Build history of the part. All positions in model axes, mm. Face numbers are marked on the shaded views. A direction names the side the tool comes from. Give positions to 0.01 mm unless a question says otherwise; leave off trailing zeros. Write each loop counter-clockwise with the first axis right and the second up, starting at its lowest first coordinate (ties: lowest second). Pieces come first, ordered by that corner, then holes. Notation, with made-up numbers: (2.25, 83) -> (28.25, 83) arc R21 ccw to (28.25, 109) -> close; hole circle Ø4 at (68, -30). An arc over 180 degrees is marked (long way). Put each result on its own line as item: value.
from build123d import *

# Parameters (mm, degrees)
SKETCH1_W           = 126
SKETCH1_H           = 68
BOSS_EXTRUDE1_DEPTH = 40
SKETCH2_W           = 117
SKETCH2_H           = 59
CUT_EXTRUDE1_DEPTH  = 38
SKETCH3_W           = 126
SKETCH3_H           = 68
SKETCH3_W_2         = 117.4
SKETCH3_H_2         = 59.4
CUT_EXTRUDE2_DEPTH  = 38
SKETCH4_R           = 10
CUT_EXTRUDE3_DEPTH  = 38
SKETCH6_R           = 1.6
CUT_EXTRUDE4_DEPTH  = 41


with BuildPart() as part:
    # Sketch1 → Boss-Extrude1 (new body)
    with BuildSketch(Plane(origin=(0, 0, 0), x_dir=(1, 0, 0), z_dir=(0, 1, 0))):
        Rectangle(SKETCH1_W, SKETCH1_H)
    extrude(amount=BOSS_EXTRUDE1_DEPTH)

    # Sketch2 → Cut-Extrude1 (cut)
    with BuildSketch(Plane(origin=(0, 40, 0), x_dir=(1, 0, 0), z_dir=(0, 1, 0))):
        Rectangle(SKETCH2_W, SKETCH2_H)
    extrude(amount=-CUT_EXTRUDE1_DEPTH, mode=Mode.SUBTRACT)

    # Sketch3 → Cut-Extrude2 (cut)
    with BuildSketch(Plane.XZ):
        Rectangle(SKETCH3_W, SKETCH3_H)
        Rectangle(SKETCH3_W_2, SKETCH3_H_2, mode=Mode.SUBTRACT)
    extrude(amount=-CUT_EXTRUDE2_DEPTH, mode=Mode.SUBTRACT)

    # Sketch4 → Cut-Extrude3 (cut)
    with BuildSketch(Plane.ZY.offset(63)):
        with Locations((0, 40)):
            Circle(SKETCH4_R)
    extrude(amount=-CUT_EXTRUDE3_DEPTH, mode=Mode.SUBTRACT)

    # Sketch6 → Cut-Extrude4 (cut, through all)
    with BuildSketch(Plane.XZ):
        with Locations((61, 15)):
            Circle(SKETCH6_R)
        with Locations((-61, 18)):
            Circle(SKETCH6_R)
        with Locations((-61, -18)):
            Circle(SKETCH6_R)
        with Locations((61, -15)):
            Circle(SKETCH6_R)
        with Locations((-21, 32)):
            Circle(SKETCH6_R)
        with Locations((-21, -32)):
            Circle(SKETCH6_R)
        with Locations((29, 32)):
            Circle(SKETCH6_R)
        with Locations((29, -32)):
            Circle(SKETCH6_R)
    extrude(amount=-CUT_EXTRUDE4_DEPTH, mode=Mode.SUBTRACT)


solid = part.part
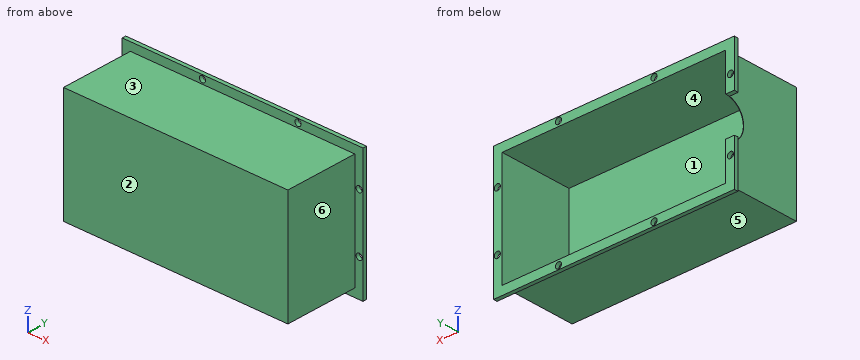
1) Slice it at D-D (x = -61). Write the cut outline in (y, z), plus the area to 3 significant figures.
Filled sheet:
outline: (38, -34) -> (40, -34) -> (40, -19.6) -> (38, -19.6) -> close; (38, -16.4) -> (40, -16.4) -> (40, -10) arc R10 cw to (38, -9.8) -> close; (38, 9.8) arc R10 cw to (40, 10) -> (40, 16.4) -> (38, 16.4) -> close; (38, 19.6) -> (40, 19.6) -> (40, 34) -> (38, 34) -> close
area: 83.5 mm2
2) Slice it at B-B (x = -21). Write the cut outline in (y, z).
Filled sheet:
outline: (0, -29.7) -> (38, -29.7) -> (38, -30.4) -> (40, -30.4) -> (40, -29.5) -> (2, -29.5) -> (2, 29.5) -> (40, 29.5) -> (40, 30.4) -> (38, 30.4) -> (38, 29.7) -> (0, 29.7) -> close; (38, -34) -> (40, -34) -> (40, -33.6) -> (38, -33.6) -> close; (38, 33.6) -> (40, 33.6) -> (40, 34) -> (38, 34) -> close
3) Wall check: L1, parallel to Z at x = 61, y = 39.1; L2, parallel to Z at x = -21, y = 39.05; L3, parallel to Z at x = 38.5, y = 17.5. Give the ranges that are in metal, low to high.
Filled sheet:
L1: -34 to -16.6, -13.4 to 13.4, 16.6 to 34
L2: -34 to -33.6, -30.4 to -29.5, 29.5 to 30.4, 33.6 to 34
L3: -29.7 to -29.5, 29.5 to 29.7
4) Slice it at A-A (z = 32). Write the cut outline in (x, y).
Filled sheet:
outline: (-63, 38) -> (-22.6, 38) -> (-22.6, 40) -> (-63, 40) -> close; (-19.4, 38) -> (27.4, 38) -> (27.4, 40) -> (-19.4, 40) -> close; (30.6, 38) -> (63, 38) -> (63, 40) -> (30.6, 40) -> close
5) Pull direction Z, two halves, no side cores. Call the marked faces 1, 2 and 3: released by +Z, released by -Z, zero draft, split by the parting line, or undercut.
Filled sheet:
face 1: undercut
face 2: zero draft
face 3: released by +Z
6) Tool access for the marked faces 4, 5 and 6: list every direction of +Z, -Z, +X, -X, +Y, -Y with a clear straight run to the whole face (end or side of a thin tool).
Filled sheet:
face 4: +Y
face 5: -Z, +X, -X, -Y
face 6: +Z, -Z, +X, -Y
7) Slice it at C-C (y = 28). Write the cut outline in (x, z), plus the area to 3 significant figures.
Filled sheet:
outline: (-58.7, -29.7) -> (58.7, -29.7) -> (58.7, 29.7) -> (-58.7, 29.7) -> close; hole (-58.5, -29.5) -> (58.5, -29.5) -> (58.5, 29.5) -> (-58.5, 29.5) -> close
area: 70.6 mm2
8) Pin check, flat tips, straight feed: pin 1 (11.5 mm diameter, centred on x = -16.5, y = 11, fed in from +Z); pin 2 (8 mm diameter, centred on x = 40.5, z = -18, fed in from +Y); pin 3 (20.5 mm diameter, centred on x = -7, z = -17, fed in from -Y); pin 4 (1.5 mm diameter, centred on x = 19.5, y = 32, fed in from -Z). Stop position of each tip, or through.
Filled sheet:
pin 1: z = 29.7
pin 2: y = 2
pin 3: y = 0
pin 4: z = -29.7
